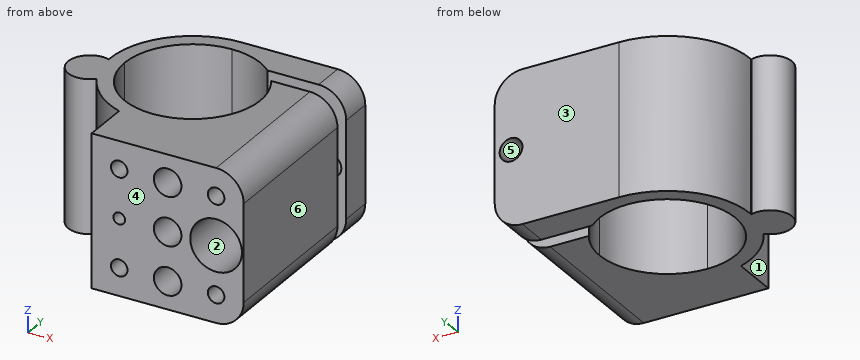
from build123d import *

# Parameters (mm, degrees)
SKETCH1_W           = 28
SKETCH1_H           = 28
BOSS_EXTRUDE1_DEPTH = 10.5
BOSS_EXTRUDE3_DEPTH = 28
SKETCH3_R           = 4
BOSS_EXTRUDE4_DEPTH = 28
BOSS_EXTRUDE5_START = -28
BOSS_EXTRUDE5_DEPTH = 28
CUT_EXTRUDE1_DEPTH  = 56.774700458
BOSS_EXTRUDE6_START = -28
BOSS_EXTRUDE6_DEPTH = 28
SKETCH8_R           = 2.1
CUT_EXTRUDE2_DEPTH  = 12.75
SKETCH1_4_R         = 1.524
SKETCH1_4_R_2       = 1.0795
CUT_EXTRUDE3_DEPTH  = 5.2
SKETCH1_5_R         = 2.54
CUT_EXTRUDE4_DEPTH  = 9.5
SKETCH1_6_R         = 4.7625
CUT_EXTRUDE5_DEPTH  = 14.5
FILLET1_R           = 5.08
FILLET2_R           = 5.08
FILLET3_R           = 5.08
FILLET4_R           = 5.08


with BuildPart() as part:
    # Sketch1 → Boss-Extrude1 (new body)
    with BuildSketch(Plane(origin=(0, 0, 0), x_dir=(1, 0, 0), z_dir=(0, 1, 0))):
        Rectangle(SKETCH1_W, SKETCH1_H)
    extrude(amount=BOSS_EXTRUDE1_DEPTH)

    # Sketch2 → Boss-Extrude3 (add)
    with BuildSketch(Plane(origin=(0, 0, -14), x_dir=(-1, 0, 0), z_dir=(0, 0, -1))):
        with BuildLine():
            ThreePointArc((21.39, 23), (17.728834765, 14.161165235), (8.89, 10.5))
            Line((8.89, 10.5), (14, 10.5))
            Line((14, 10.5), (14, 8.631618045))
            ThreePointArc((14, 8.631618045), (21.34973515, 14.206962982), (24.14, 23))
            Line((24.14, 23), (21.39, 23))
        make_face()
        with BuildLine():
            Line((8.89, 10.5), (8.89, 7.75))
            ThreePointArc((8.89, 7.75), (11.482747113, 7.972020681), (14, 8.631618045))
            Line((14, 8.631618045), (14, 10.5))
            Line((14, 10.5), (8.89, 10.5))
        make_face()
        with BuildLine():
            Line((0.154297395, 10.5), (8.89, 10.5))
            ThreePointArc((8.89, 10.5), (0.051165235, 14.161165235), (-3.61, 23))
            Line((-3.61, 23), (-6.36, 23))
            ThreePointArc((-6.36, 23), (-4.63371925, 15.952197673), (0.154297395, 10.5))
        make_face()
        with BuildLine():
            ThreePointArc((0.154297395, 10.5), (4.310835229, 8.453737593), (8.89, 7.75))
            Line((8.89, 7.75), (8.89, 10.5))
            Line((8.89, 10.5), (0.154297395, 10.5))
        make_face()
        with BuildLine():
            ThreePointArc((8.89, 35.5), (17.728834765, 31.838834765), (21.39, 23))
            Line((21.39, 23), (24.14, 23))
            ThreePointArc((24.14, 23), (19.673378413, 33.783378413), (8.89, 38.25))
            Line((8.89, 38.25), (8.89, 35.5))
        make_face()
        with BuildLine():
            Line((-6.36, 23), (-3.61, 23))
            ThreePointArc((-3.61, 23), (0.051165235, 31.838834765), (8.89, 35.5))
            Line((8.89, 35.5), (8.89, 38.25))
            ThreePointArc((8.89, 38.25), (-1.893378413, 33.783378413), (-6.36, 23))
        make_face()
    extrude(amount=-BOSS_EXTRUDE3_DEPTH)

    # Sketch3 → Boss-Extrude4 (add)
    with BuildSketch(Plane.XY.offset(14)):
        with Locations((-25.389704171, 18.914002035)):
            Circle(SKETCH3_R)
    extrude(amount=-BOSS_EXTRUDE4_DEPTH)

    # Sketch5 → Boss-Extrude5 (add)
    with BuildSketch(Plane.XY.offset(14).offset(BOSS_EXTRUDE5_START)):
        with BuildLine():
            ThreePointArc((4.905379661, 29.5), (5.846431624, 19.075706053), (-0.154297395, 10.5))
            Line((-0.154297395, 10.5), (14, 10.5))
            Line((14, 10.5), (14, 29.5))
            Line((14, 29.5), (4.905379661, 29.5))
        make_face()
    extrude(amount=BOSS_EXTRUDE5_DEPTH)

    # Sketch6 → Cut-Extrude1 (cut, through all)
    with BuildSketch(Plane.XY.offset(14)):
        with BuildLine():
            Line((14, 29.5), (14, 32.25))
            Line((14, 32.25), (-0.48241414, 32.25))
            ThreePointArc((-0.48241414, 32.25), (0.750888241, 30.956335459), (1.787078252, 29.5))
            Line((1.787078252, 29.5), (14, 29.5))
        make_face()
    extrude(amount=-CUT_EXTRUDE1_DEPTH, mode=Mode.SUBTRACT)

    # Sketch7 → Boss-Extrude6 (add)
    with BuildSketch(Plane.XY.offset(14).offset(BOSS_EXTRUDE6_START)):
        with BuildLine():
            Line((14, 38.25), (-8.89, 38.25))
            ThreePointArc((-8.89, 38.25), (-3.444771469, 37.244717837), (1.282556587, 34.361408032))
            Line((1.282556587, 34.361408032), (6.806, 32.25))
            Line((6.806, 32.25), (14, 32.25))
            Line((14, 32.25), (14, 38.25))
        make_face()
        with BuildLine():
            Line((6.806, 32.25), (1.282556587, 34.361408032))
            ThreePointArc((1.282556587, 34.361408032), (2.308329555, 33.351807338), (3.234355653, 32.25))
            Line((3.234355653, 32.25), (6.806, 32.25))
        make_face()
    extrude(amount=BOSS_EXTRUDE6_DEPTH)

    # Sketch8 → Cut-Extrude2 (cut)
    with BuildSketch(Plane(origin=(0, 38.25, 0), x_dir=(1, 0, 0), z_dir=(0, 1, 0))):
        with Locations(Location((11, 0, 0), (0, 0, 270))):
            Circle(SKETCH8_R)
    extrude(amount=-CUT_EXTRUDE2_DEPTH, mode=Mode.SUBTRACT)

    # Sketch1<4> → Cut-Extrude3 (cut)
    with BuildSketch(Plane(origin=(0, 0, 0), x_dir=(1, 0, 0), z_dir=(0, 1, 0))):
        with Locations(Location((-8.92, 8.92, 0), (0, 0, 270))):
            Circle(SKETCH1_4_R)
        with Locations(Location((8.92, 8.92, 0), (0, 0, 270))):
            Circle(SKETCH1_4_R)
        with Locations(Location((8.92, -8.92, 0), (0, 0, 270))):
            Circle(SKETCH1_4_R)
        with Locations(Location((-8.92, -8.92, 0), (0, 0, 270))):
            Circle(SKETCH1_4_R)
        with Locations(Location((-8.92, 0, 0), (0, 0, 270))):
            Circle(SKETCH1_4_R_2)
    extrude(amount=CUT_EXTRUDE3_DEPTH, mode=Mode.SUBTRACT)

    # Sketch1<5> → Cut-Extrude4 (cut)
    with BuildSketch(Plane(origin=(0, 0, 0), x_dir=(1, 0, 0), z_dir=(0, 1, 0))):
        with Locations(Location((0, 8.92, 0), (0, 0, 270))):
            Circle(SKETCH1_5_R)
        with Locations(Location((0, -8.92, 0), (0, 0, 270))):
            Circle(SKETCH1_5_R)
        with Locations(Location((0, 0, 0), (0, 0, 270))):
            Circle(SKETCH1_5_R)
    extrude(amount=CUT_EXTRUDE4_DEPTH, mode=Mode.SUBTRACT)

    # Sketch1<6> → Cut-Extrude5 (cut)
    with BuildSketch(Plane(origin=(0, 0, 0), x_dir=(1, 0, 0), z_dir=(0, 1, 0))):
        with Locations(Location((8.92, 0, 0), (0, 0, 90))):
            Circle(SKETCH1_6_R)
    extrude(amount=CUT_EXTRUDE5_DEPTH, mode=Mode.SUBTRACT)

    # Fillet1
    fillet1_edges = [part.edges().sort_by_distance(p)[0] for p in [
        (14, 14.75, 14),
    ]]
    fillet(fillet1_edges, radius=FILLET1_R)

    # Fillet2
    fillet2_edges = [part.edges().sort_by_distance(p)[0] for p in [
        (14, 35.25, 14),
    ]]
    fillet(fillet2_edges, radius=FILLET2_R)

    # Fillet3
    fillet3_edges = [part.edges().sort_by_distance(p)[0] for p in [
        (14, 35.25, -14),
    ]]
    fillet(fillet3_edges, radius=FILLET3_R)

    # Fillet4
    fillet4_edges = [part.edges().sort_by_distance(p)[0] for p in [
        (14, 14.75, -14),
    ]]
    fillet(fillet4_edges, radius=FILLET4_R)


solid = part.part
Input: part model. Units: mm. Frame: model coordinates. Face numbers are marked on the shaded views. A direction names the side the tool comes from. Give positions to 0.01 mm unless a question says otherwise; leave off trailing zeros. Write each loop counter-clockwise with the first axis right and the second up, starting at its lowest first coordinate (ties: lowest second). Pieces come first, ordered by that corner, then holes.
Q1. Section D-D, the plane x = 11. Output: boundary loops of the cut face in (y, z), plus the area to 3 significant figures.
Q2. First-contact query: P1, Ø12, axis at x = -18.5, z = 2, coming from the +Y side; P2, Ø0.9, axis at x = 8, z = 9, coming from the -Y side; P3, Ø9.5, axis at y = 3.5, z = 3.5, coming from the -X side; P4, Ø1, axis at x = -14.5, y = 31.5, coming from the -Z side. Flat tips, straight axial feed; report the tip coordinate or a pass-through.
Q3. Section A-A, the plane y = 27.5. Output: boundary loops of the cut face in (x, z).
Q4. Section C-C, the plane y = 3.5. State how many separate pieces and enclosed holes the cut face has, plus the area to 3 significant figures.
Q5. Pull-direction query (X, two-part tool) for the marked faces 4, 5 and 6; classes: pulls with the +X half, pulls with the -X half, needs draft (parallel to the pull), parting line crosses it, or undercut.
Q6. Section B-B, the plane z = 5.75. Output: boundary loops of the cut face in (x, y).
Q7. Material intervals for probe 1 along X at (y, z) = (2.5, -8.92); probe 2 along X at (y, z) = (5.75, 0); probe 3 along Y at (x, z) = (2, 7), sorted ascending.
Q8. Set-up query: the marked faces 1, 2 and 3. Return all of +Z, -Z, +X, -X, +Y, -Y with unobstructed straight access to the full face (end or side cutting, diameter ignored); none if empty.
Filled in:
1. outline: (0, -13.55) - (29.5, -13.55) - (29.5, -2.1) - (25.5, -2.1) - (25.5, 2.1) - (29.5, 2.1) - (29.5, 13.55) - (0, 13.55) - (0, 4.28) - (14.5, 4.28) - (14.5, -4.28) - (0, -4.28) - close; (32.25, -13.55) - (38.25, -13.55) - (38.25, -2.1) - (32.25, -2.1) - close; (32.25, 2.1) - (38.25, 2.1) - (38.25, 13.55) - (32.25, 13.55) - close
1. area: 796 mm2
2. P1: stops at y = 37.82
2. P2: stops at y = 5.2
2. P3: stops at x = -14
2. P4: passes through
3. outline: (-23.46, -14) - (-20.55, -14) - (-20.55, 14) - (-23.46, 14) - close; (2.77, -14) - (8.92, -14) arc R5.08 ccw to (14, -8.92) - (14, 8.92) arc R5.08 ccw to (8.92, 14) - (2.77, 14) - close; hole circle Ø4.2 at (11, 0)
4. separate pieces: 1
4. enclosed holes: 9
4. area: 608 mm2
5. face 4: needs draft
5. face 5: undercut
5. face 6: pulls with the +X half
6. outline: (-24.14, 22.71) arc R4 ccw (long way) to (-22.51, 16.14) arc R15.25 ccw to (-14, 8.63) - (-14, 0) - (14, 0) - (14, 29.5) - (1.79, 29.5) arc R12.5 cw (long way) to (-0.48, 32.25) - (14, 32.25) - (14, 38.25) - (-8.89, 38.25) arc R15.25 ccw to start
7. probe 1: x = -14 to -10.44, -7.4 to -2.54, 2.54 to 7.4, 10.44 to 14
7. probe 2: x = -14 to -2.54, 2.54 to 4.16, 13.68 to 14
7. probe 3: y = 0 to 16.86, 29.14 to 29.5, 32.25 to 38.25
8. face 1: +Z, -Z, -X, -Y
8. face 2: -Y
8. face 3: +Z, -Z, +X, -X, +Y
